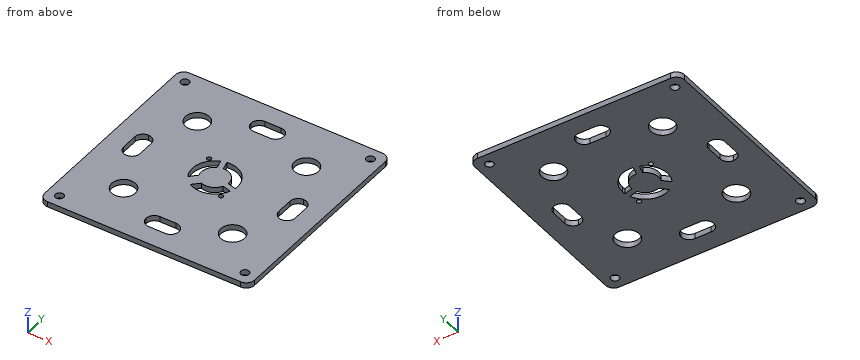
```python
from build123d import *

# Parameters (mm, degrees)
SKETCH_1_R          = 1.5
SKETCH_1_R_2        = 4.35
EXTRUDE_1_DEPTH     = 2
SKETCH_3_R          = 0.82
CUT_EXTRUDE_2_DEPTH = 10
EXTRUDE_START       = -2
EXTRUDE_2_DEPTH     = 2
FILLET_1_R          = 3


with BuildPart() as part:
    # 草圖1 → 填料-伸長1 (new body)
    with BuildSketch(Plane.XY):
        with BuildLine():
            Line((-35.45, 38.45), (35.45, 38.45))
            ThreePointArc((35.45, 38.45), (37.571320344, 37.571320344), (38.45, 35.45))
            Line((38.45, 35.45), (38.45, -35.45))
            ThreePointArc((38.45, -35.45), (37.571320344, -37.571320344), (35.45, -38.45))
            Line((35.45, -38.45), (-35.45, -38.45))
            ThreePointArc((-35.45, -38.45), (-37.571320344, -37.571320344), (-38.45, -35.45))
            Line((-38.45, -35.45), (-38.45, 35.45))
            ThreePointArc((-38.45, 35.45), (-37.571320344, 37.571320344), (-35.45, 38.45))
        make_face()
        with Locations((-34, 34)):
            Circle(SKETCH_1_R, mode=Mode.SUBTRACT)
        with Locations((34, 34)):
            Circle(SKETCH_1_R, mode=Mode.SUBTRACT)
        with Locations((34, -34)):
            Circle(SKETCH_1_R, mode=Mode.SUBTRACT)
        with Locations((-34, -34)):
            Circle(SKETCH_1_R, mode=Mode.SUBTRACT)
        with Locations((-20, 20)):
            Circle(SKETCH_1_R_2, mode=Mode.SUBTRACT)
        with Locations((20, 20)):
            Circle(SKETCH_1_R_2, mode=Mode.SUBTRACT)
        with Locations((-20, -20)):
            Circle(SKETCH_1_R_2, mode=Mode.SUBTRACT)
        with Locations((20, -20)):
            Circle(SKETCH_1_R_2, mode=Mode.SUBTRACT)
        with BuildLine():
            Line((-18.5, 31.45), (18.5, 31.45))
            Line((18.5, 31.45), (18.5, 26.837397166))
            ThreePointArc((18.5, 26.837397166), (15.050252532, 24.949747468), (13.162602834, 21.5))
            Line((13.162602834, 21.5), (-13.162602834, 21.5))
            ThreePointArc((-13.162602834, 21.5), (-15.050252532, 24.949747468), (-18.5, 26.837397166))
            Line((-18.5, 26.837397166), (-18.5, 31.45))
        make_face(mode=Mode.SUBTRACT)
        with BuildLine():
            Line((-31.45, 18.5), (-31.45, -18.5))
            Line((-31.45, -18.5), (-26.837397166, -18.5))
            ThreePointArc((-26.837397166, -18.5), (-24.949747468, -15.050252532), (-21.5, -13.162602834))
            Line((-21.5, -13.162602834), (-21.5, 13.162602834))
            ThreePointArc((-21.5, 13.162602834), (-24.949747468, 15.050252532), (-26.837397166, 18.5))
            Line((-26.837397166, 18.5), (-31.45, 18.5))
        make_face(mode=Mode.SUBTRACT)
        with BuildLine():
            Line((26.837397166, 18.5), (31.45, 18.5))
            Line((31.45, 18.5), (31.45, -18.5))
            Line((31.45, -18.5), (26.837397166, -18.5))
            ThreePointArc((26.837397166, -18.5), (24.949747468, -15.050252532), (21.5, -13.162602834))
            Line((21.5, -13.162602834), (21.5, 13.162602834))
            ThreePointArc((21.5, 13.162602834), (24.949747468, 15.050252532), (26.837397166, 18.5))
        make_face(mode=Mode.SUBTRACT)
        with BuildLine():
            Line((-18.5, -31.45), (-18.5, -26.837397166))
            ThreePointArc((-18.5, -26.837397166), (-15.050252532, -24.949747468), (-13.162602834, -21.5))
            Line((-13.162602834, -21.5), (13.162602834, -21.5))
            ThreePointArc((13.162602834, -21.5), (15.050252532, -24.949747468), (18.5, -26.837397166))
            Line((18.5, -26.837397166), (18.5, -31.45))
            Line((18.5, -31.45), (-18.5, -31.45))
        make_face(mode=Mode.SUBTRACT)
    extrude(amount=EXTRUDE_1_DEPTH)

    # 草圖3 → 除料-伸長2 (cut)
    with BuildSketch(Plane.XY.offset(2)):
        with BuildLine():
            Line((-7.073829274, -4.245402149), (-4.654583912, -1.826156787))
            ThreePointArc((-4.654583912, -1.826156787), (-4.667257292, 1.793518711), (-2.233875019, 4.473231762))
            Line((-2.233875019, 4.473231762), (-3.085438902, 7.651311442))
            ThreePointArc((-3.085438902, 7.651311442), (-7.822124458, 2.622378494), (-7.073829274, -4.245402149))
        make_face()
        with BuildLine():
            Line((-1.15358725, 8.168949532), (-0.302023366, 4.990869853))
            ThreePointArc((-0.302023366, 4.990869853), (3.427089375, 3.640749705), (5, 0))
            ThreePointArc((5, 0), (4.997716942, -0.151080668), (4.990869853, -0.302023366))
            Line((4.990869853, -0.302023366), (8.168949532, -1.15358725))
            ThreePointArc((8.168949532, -1.15358725), (8.229712438, -0.578215514), (8.25, 0))
            ThreePointArc((8.25, 0), (5.410425362, 6.228145583), (-1.15358725, 8.168949532))
        make_face()
        with BuildLine():
            ThreePointArc((4.473231762, -2.233875019), (1.793518711, -4.667257292), (-1.826156787, -4.654583912))
            Line((-1.826156787, -4.654583912), (-4.245402149, -7.073829274))
            ThreePointArc((-4.245402149, -7.073829274), (2.622378494, -7.822124458), (7.651311442, -3.085438902))
            Line((7.651311442, -3.085438902), (4.473231762, -2.233875019))
        make_face()
        with Locations((6.717514421, -6.717514421)):
            Circle(SKETCH_3_R)
        with Locations((-6.717514421, 6.717514421)):
            Circle(SKETCH_3_R)
    extrude(amount=-CUT_EXTRUDE_2_DEPTH, mode=Mode.SUBTRACT)

    # 草圖4 → 填料-伸長2 (add)
    with BuildSketch(Plane.XY.offset(2).offset(EXTRUDE_START)):
        with BuildLine():
            Line((-31.45, -6), (-31.45, -18.5))
            Line((-31.45, -18.5), (-26.837397166, -18.5))
            ThreePointArc((-26.837397166, -18.5), (-24.949747468, -15.050252532), (-21.5, -13.162602834))
            Line((-21.5, -13.162602834), (-21.5, 13.162602834))
            ThreePointArc((-21.5, 13.162602834), (-24.949747468, 15.050252532), (-26.837397166, 18.5))
            Line((-26.837397166, 18.5), (-31.45, 18.5))
            Line((-31.45, 18.5), (-31.45, 6))
            Line((-31.45, 6), (-25.45, 6))
            Line((-25.45, 6), (-25.45, -6))
            Line((-25.45, -6), (-31.45, -6))
        make_face()
        with BuildLine():
            Line((-6, 31.45), (-18.5, 31.45))
            Line((-18.5, 31.45), (-18.5, 26.837397166))
            ThreePointArc((-18.5, 26.837397166), (-15.050252532, 24.949747468), (-13.162602834, 21.5))
            Line((-13.162602834, 21.5), (13.162602834, 21.5))
            ThreePointArc((13.162602834, 21.5), (15.050252532, 24.949747468), (18.5, 26.837397166))
            Line((18.5, 26.837397166), (18.5, 31.45))
            Line((18.5, 31.45), (6, 31.45))
            Line((6, 31.45), (6, 25.45))
            Line((6, 25.45), (-6, 25.45))
            Line((-6, 25.45), (-6, 31.45))
        make_face()
        with BuildLine():
            Line((31.45, 6), (31.45, 18.5))
            Line((31.45, 18.5), (26.837397166, 18.5))
            ThreePointArc((26.837397166, 18.5), (24.949747468, 15.050252532), (21.5, 13.162602834))
            Line((21.5, 13.162602834), (21.5, -13.162602834))
            ThreePointArc((21.5, -13.162602834), (24.949747468, -15.050252532), (26.837397166, -18.5))
            Line((26.837397166, -18.5), (31.45, -18.5))
            Line((31.45, -18.5), (31.45, -6))
            Line((31.45, -6), (25.45, -6))
            Line((25.45, -6), (25.45, 6))
            Line((25.45, 6), (31.45, 6))
        make_face()
        with BuildLine():
            Line((6, -31.45), (18.5, -31.45))
            Line((18.5, -31.45), (18.5, -26.837397166))
            ThreePointArc((18.5, -26.837397166), (15.050252532, -24.949747468), (13.162602834, -21.5))
            Line((13.162602834, -21.5), (-13.162602834, -21.5))
            ThreePointArc((-13.162602834, -21.5), (-15.050252532, -24.949747468), (-18.5, -26.837397166))
            Line((-18.5, -26.837397166), (-18.5, -31.45))
            Line((-18.5, -31.45), (-6, -31.45))
            Line((-6, -31.45), (-6, -25.45))
            Line((-6, -25.45), (6, -25.45))
            Line((6, -25.45), (6, -31.45))
        make_face()
    extrude(amount=EXTRUDE_2_DEPTH)

    # 圓角1
    fillet_1_edges = [part.edges().sort_by_distance(p)[0] for p in [
        (-25.45, -6, 1),
        (-31.45, -6, 1),
        (-25.45, 6, 1),
        (-31.45, 6, 1),
        (6, 31.45, 1),
        (6, 25.45, 1),
        (-6, 31.45, 1),
        (-6, 25.45, 1),
        (31.45, 6, 1),
        (25.45, 6, 1),
        (31.45, -6, 1),
        (25.45, -6, 1),
        (-6, -31.45, 1),
        (-6, -25.45, 1),
        (6, -31.45, 1),
        (6, -25.45, 1),
    ]]
    fillet(fillet_1_edges, radius=FILLET_1_R - 0.0001)  # a hair under: the kernel refuses the full size


solid = part.part
```
Geometry check sheet. Reference: the model listing, model coordinates, mm. Coordinates: 2 decimals unless noted, no trailing zeros. Loops run counter-clockwise (first coordinate to the right, second up) from the corner with the lowest first, then second, coordinate; pieces in that order, holes last.
Item 1: Go/stop test with a flat-tipped pin: pin 1 Ø2.5 at (x, y) = (34, 34) entering from +Z. Record where the tip stops, or that it passes through.
Item 2: Thickness scan on line 1 (Y direction, x = -20, z = 0.7); line 2 (X direction, y = -4, z = 1.5); line 3 (Y direction, x = -34, z = 0.8). Record the ranges inside material, lowest first.
Item 3: Sectioned sample at D-D, the plane z = 1. Count the separate pieces of the cut face and the enclosed holes in it, then the cut area to 3 significant figures.
Item 4: Sectioned sample at B-B, the plane x = 34. Record the boundary of the cut face in (y, z), then the cut area to 3 significant figures.
Item 5: Sectioned sample at C-C, the plane x = -26.5. Record the boundary of the cut face in (y, z).
Item 6: Sectioned sample at A-A, the plane y = -20. Record the boundary of the cut face in (x, z), then the cut area to 3 significant figures.
Check result:
1. pin 1: passes through
2. line 1: y = -38.45 to -24.35, -15.65 to 15.65, 24.35 to 38.45
2. line 2: x = -38.45 to -31.28, -25.62 to -7.22, -6.83 to 3, 7.22 to 25.62, 31.28 to 38.45
2. line 3: y = -38.45 to -35.5, -32.5 to 32.5, 35.5 to 38.45
3. separate pieces: 1
3. enclosed holes: 17
3. area: 5,270 mm2
4. outline: (-38.45, 0) - (-35.5, 0) - (-35.5, 2) - (-38.45, 2) - close; (-32.5, 0) - (32.5, 0) - (32.5, 2) - (-32.5, 2) - close; (35.5, 0) - (38.45, 0) - (38.45, 2) - (35.5, 2) - close
4. area: 142 mm2
5. outline: (-38.45, 0) - (-5.28, 0) - (-5.28, 2) - (-38.45, 2) - close; (5.28, 0) - (38.45, 0) - (38.45, 2) - (5.28, 2) - close
6. outline: (-38.45, 0) - (-24.35, 0) - (-24.35, 2) - (-38.45, 2) - close; (-15.65, 0) - (15.65, 0) - (15.65, 2) - (-15.65, 2) - close; (24.35, 0) - (38.45, 0) - (38.45, 2) - (24.35, 2) - close
6. area: 119 mm2
